Input: part model. Units: mm. Frame: model coordinates. Round coordinates to 2 decimals unless told otherwise and drop trailing zeros. Write each loop counter-clockwise with the first axis right and the second up, starting at its lowest first coordinate (ties: lowest second). Pieces come first, ordered by that corner, then holes. Notation, with made-up numbers: (44, 50) -> (86, 50) arc R21 ccw to (86, 55) -> close; hole circle Ø11 at (73, -21). An arc over 180 degrees is marked (long way). Use CSV: the item, a comma, the result in double quotes.
```python
from build123d import *

# Parameters (mm, degrees)
F1_DEPTH = 1524
F2_R     = 3.175
F3_DEPTH = 381


with BuildPart() as f1:
    # F0 (on Front) → F1 (new body)
    with BuildSketch(Plane.XZ):
        with BuildLine():
            Line((-12.7, 81.567227), (-13.208, 84.829916))
            ThreePointArc((-13.208, 84.829916), (0, -85.852), (13.208, 84.829916))
            Line((13.208, 84.829916), (12.7, 81.567227))
            ThreePointArc((12.7, 81.567227), (0, -82.55), (-12.7, 81.567227))
        make_face()
    extrude(amount=-F1_DEPTH)

    # F2 (on Top) → F3 (cut, symmetric)
    with BuildSketch(Plane.XY):
        with Locations((0, 50.8)):
            Circle(F2_R)
    extrude(amount=F3_DEPTH, both=True, mode=Mode.SUBTRACT)


solid = f1.part
```
Item 1: Section query B-B on x = -38.5. Return the cut outline in (y, z).
Worked answers:
outline,"(0, -76.74) -> (1524, -76.74) -> (1524, -73.02) -> (0, -73.02) -> close; (0, 73.02) -> (1524, 73.02) -> (1524, 76.74) -> (0, 76.74) -> close"
Item 2: Section query A-A on z = 0. Return the cut outline in (x, y), plus the area to 3 significant figures.
Worked answers:
outline,"(-85.85, 0) -> (-82.55, 0) -> (-82.55, 1524) -> (-85.85, 1524) -> close; (82.55, 0) -> (85.85, 0) -> (85.85, 1524) -> (82.55, 1524) -> close"
area,"10,100 mm²"
Item 3: First-contact query: pin 1 Ø8 at (x, y) = (58.5, 221.5) entering from +Z; pin 2 Ø2 at (x, y) = (-54, 958) entering from -Z; pin 3 Ø4 at (x, y) = (0, 50.8) entering from -Z; pin 4 Ø10 at (y, z) = (476.5, 16.5) entering from +X. Flat tips, straight axial feed; report the tip coordinate or a pass-through.
Worked answers:
pin 1,"stops at z = 66.33"
pin 2,"stops at z = -67.54"
pin 3,"passes through"
pin 4,"stops at x = 85.08"
Item 4: Line query: line 1 (Y direction, x = 0, z = -83.85) (3 decimals); line 2 (X direction, y = 1180.5, z = -3); line 3 (Z direction, x = 0, y = 1148.5). Output: solid intervals per line, ascending.
Worked answers:
line 1,"y = 0 to 47.625, 53.975 to 1524"
line 2,"x = -85.8 to -82.5, 82.5 to 85.8"
line 3,"z = -85.85 to -82.55"
Item 5: Pull-direction query (Z, two-part tool) for faces 1 (the face through (-3.589, 751.332, -85.777)), 2 (the face through (-83, 0, 0)), 3 (the face through (3.451, 751.332, -82.478)); classes: +Z half, -Z half, draft (parallel to the pull), parting line (faces both ways), or undercut.
Worked answers:
face 1,"parting line"
face 2,"draft"
face 3,"undercut"
Item 6: Section query C-C on y = 1164. Return the cut outline in (x, z), plus the area to 3 significant figures.
Worked answers:
outline,"(-13.21, 84.83) arc R85.85 ccw (long way) to (13.21, 84.83) -> (12.7, 81.57) arc R82.55 cw (long way) to (-12.7, 81.57) -> close"
area,"1,660 mm²"
